Part print with two shaded views. Sizes in mm from the minimum x, y, z corner. A direction names the side the tool comes from. Round coordinates to 2 decimals unless told otherwise and drop trailing zeros. Loops run counter-clockwise (first coordinate to the right, second up) from the corner with the lowest first, then second, coordinate; pieces in that order, holes last. Notation, with made-up numbers: (6.5, -40) - (63.5, -40) arc R9 cw to (63.5, -28) - close; hole circle Ø2 at (24, 32). An arc over 180 degrees is marked (long way). One line per question, with ' | ' between items.
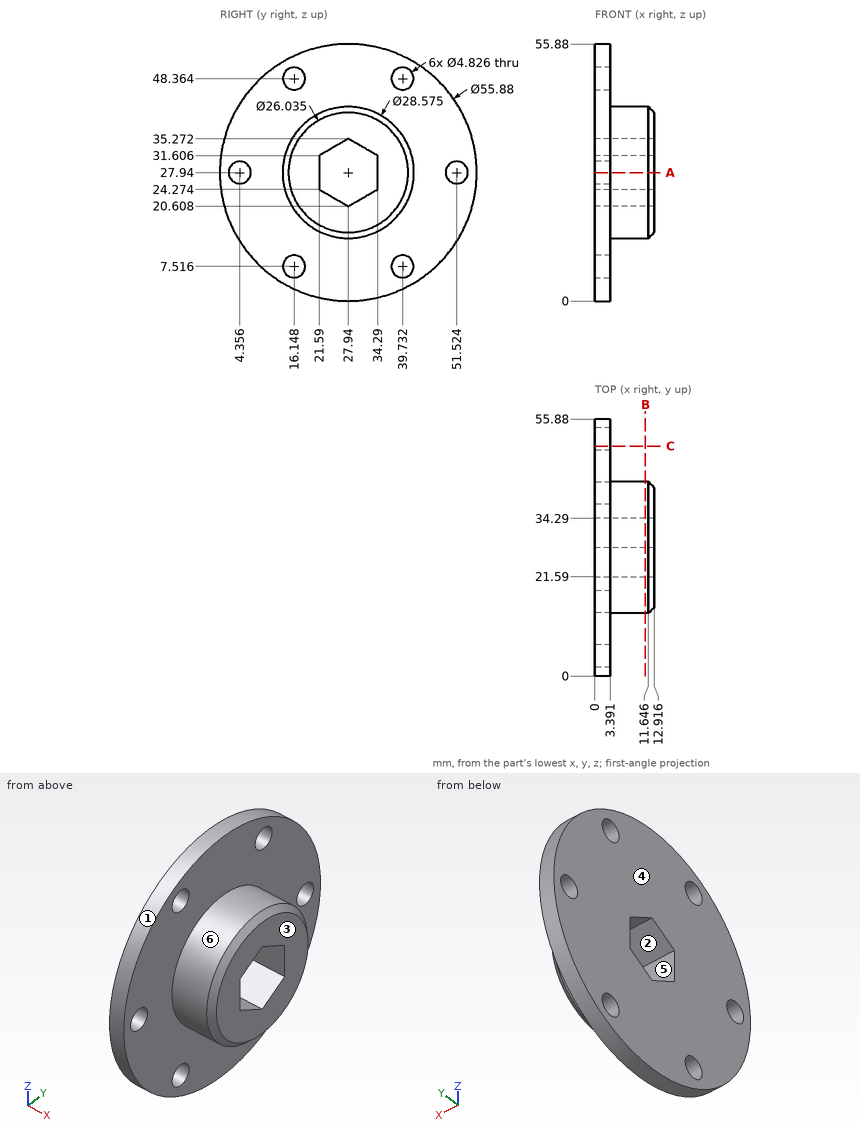
(1) Tool access for the marked faces 4, 5 and 6: list every direction of +Z, -Z, +X, -X, +Y, -Y with a clear straight run to the whole face (end or side of a thin tool).
Results found:
face 4: +Z, -Z, -X, +Y, -Y | face 5: +X, -X | face 6: +X
(2) Cut at C-C, the plane y = 50. Write the cut outline in (x, z), then the cut area to 3 significant figures.
Results found:
outline: (0, 10.79) - (3.39, 10.79) - (3.39, 26.07) - (0, 26.07) - close; (0, 29.81) - (3.39, 29.81) - (3.39, 45.09) - (0, 45.09) - close | area: 104 mm²
(3) Cut at A-A, the plane z = 27.94. Write the cut outline in (x, y), then the cut area to 3 significant figures.
Results found:
outline: (0, 0) - (3.39, 0) - (3.39, 1.94) - (0, 1.94) - close; (0, 6.77) - (3.39, 6.77) - (3.39, 13.65) - (11.65, 13.65) - (12.92, 14.92) - (12.92, 21.59) - (0, 21.59) - close; (0, 34.29) - (12.92, 34.29) - (12.92, 40.96) - (11.65, 42.23) - (3.39, 42.23) - (3.39, 49.11) - (0, 49.11) - close; (0, 53.94) - (3.39, 53.94) - (3.39, 55.88) - (0, 55.88) - close | area: 263 mm²
(4) Cut at B-B, the plane x = 11. Write the cut outline in (y, z) (1 decimal).
Results found:
outline: circle Ø28.6 at (27.9, 27.9); hole (21.6, 24.3) - (27.9, 20.6) - (34.3, 24.3) - (34.3, 31.6) - (27.9, 35.3) - (21.6, 31.6) - close
(5) Probe L1, parallel to Y at x = 1.2, z = 27.94; L2, parallel to Y at x = 4.75, z = 28; L3, parallel to X at y = 33, z = 54.5. List the from-to ranges inside material, lowest first.
Results found:
L1: y = 0 to 1.94, 6.77 to 21.59, 34.29 to 49.11, 53.94 to 55.88 | L2: y = 13.65 to 21.59, 34.29 to 42.23 | L3: x = 0 to 3.39
(6) Drop flat-ended pins along their axis: P1, Ø4.5, axis at y = 16.15, z = 48.36, coming from the -X side; P2, Ø2, axis at x = 3.5, z = 27, coming from the -Y side; P3, Ø6, axis at x = 4, z = 43, coming from the +Y side; P4, Ø3.5, axis at x = 7.5, z = 29, coming from the -Y side. Give the stop position or say it passes through.
Results found:
P1: passes through | P2: stops at y = 0 | P3: stops at y = 53.11 | P4: stops at y = 13.65
(7) Two-plate mould, pull along Y, no slides. Class the marked faces 1, 2 and 3: released by +Y, released by -Y, zero draft, split by the parting line, or undercut.
Results found:
face 1: split by the parting line | face 2: undercut | face 3: zero draft
